Drawing for the job (mm, zero at the part's lowest x, y, z). Give positions to 0.01 mm unless a question says otherwise; leave off trailing zeros. Order: outer loops, then holes, each group sorted by start corner. A loop starts at its lowest first (then second) coordinate and runs counter-clockwise, first axis right, second up. Notation, with made-up numbers: (61, -1) - (65, -1) arc R13 ccw to (65, 18) - close; hole circle Ø3 at (21.25, 84). An arc over 180 degrees is marked (long way). Use a Markdown table: item, result. Add a question column.
(1) Slice it at B-B (x = 2.5). Write the cut outline in (y, z).
(2) Slice it at D-D (x = 8.5). Write the cut outline in (y, z), then the cut area to 3 significant figures.
(3) Wall check: line 1 (X direction, y = 7.5, z = 0.15); line 2 (Y direction, x = 8, z = 0.35); line 3 (Y direction, x = 5.5, z = 0.3). Give the ranges that are in metal, low to high.
(4) Slice it at A-A (y = 6.75). Write the cut outline in (x, z).
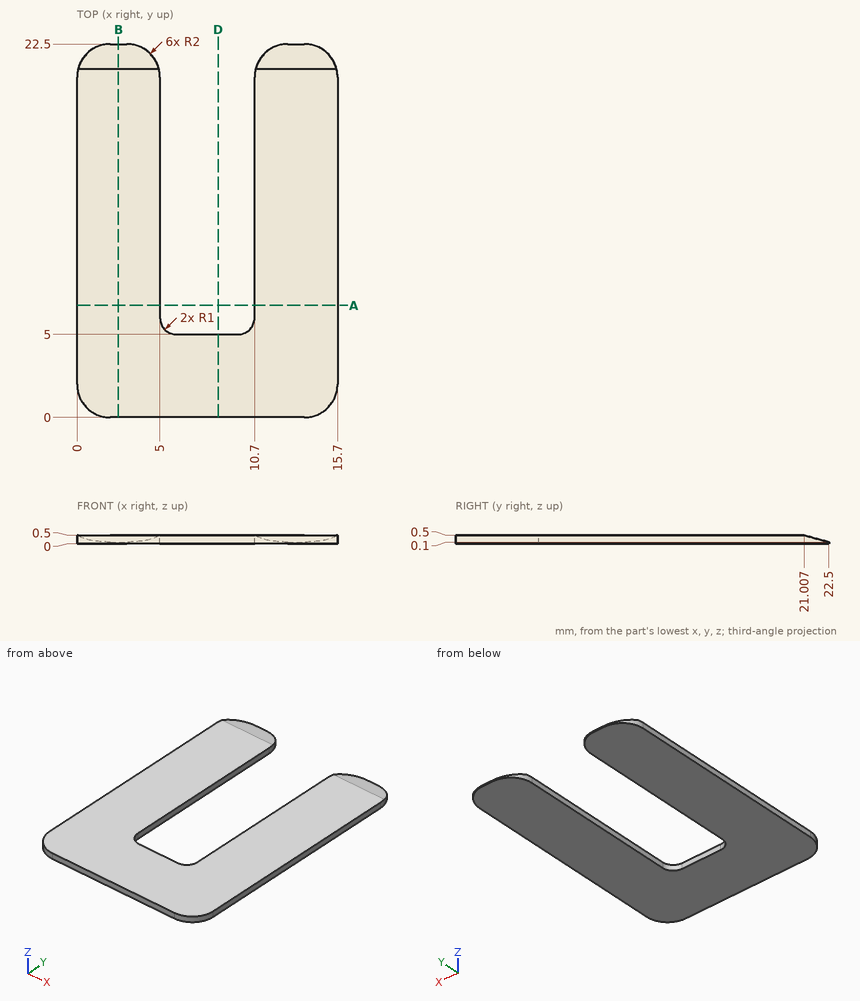
Solution:
| question | item | result |
|---|---|---|
| 1 | outline | (0, 0) - (22.5, 0) - (22.5, 0.1) - (21.01, 0.5) - (0, 0.5) - close |
| 2 | outline | (0, 0) - (5, 0) - (5, 0.5) - (0, 0.5) - close |
| 2 | area | 2.50 mm2 |
| 3 | line 1 | 0 to 5, 10.7 to 15.7 |
| 3 | line 2 | 0 to 5 |
| 3 | line 3 | 0 to 5.13 |
| 4 | outline | (0, 0) - (5, 0) - (5, 0.5) - (0, 0.5) - close; (10.7, 0) - (15.7, 0) - (15.7, 0.5) - (10.7, 0.5) - close |
